Geometry: final body of the model. Coordinates: model frame, mm. A direction names the side the tool comes from. Give positions to 0.01 mm unless a question says otherwise; leave off trailing zeros. Order: outer loops, then holes, each group sorted by start corner. A loop starts at its lowest first (then second) coordinate and runs counter-clockwise, first axis right, second up. Notation, with made-up numbers: (-39, 23) -> (16, 23) arc R20 ccw to (16, 30) -> close; hole circle Ø3 at (14.5, -15.75). An arc over 180 degrees is marked (long way). One line per item, written item: value. Start each with the question number.
```python
from build123d import *

# Parameters (mm, degrees)
EXTRUDE_1_DEPTH     = 60
SKETCH_3_R          = 2.3
CUT_EXTRUDE_1_DEPTH = 30
SKETCH_4_W          = 30
SKETCH_4_H          = 50
EXTRUDE_2_DEPTH     = 3
EXTRUDE_3_DEPTH     = 15
SKETCH_6_W          = 47.657493386
SKETCH_6_H          = 61.593201797
CUT_EXTRUDE_2_DEPTH = 30
SKETCH_7_R          = 3.2
CUT_EXTRUDE_3_DEPTH = 3


with BuildPart() as part:
    # 草图2 → 凸台-拉伸1 (new body)
    with BuildSketch(Plane(origin=(0, 0, 0), x_dir=(1, 0, 0), z_dir=(0, 1, 0))):
        with BuildLine():
            Line((-4, 6), (4, 6))
            ThreePointArc((4, 6), (10, 0), (4, -6))
            Line((4, -6), (-4, -6))
            ThreePointArc((-4, -6), (-10, 0), (-4, 6))
        make_face()
        with BuildLine():
            Line((-2.5, 4.05), (2.5, 4.05))
            ThreePointArc((2.5, 4.05), (6.55, 0), (2.5, -4.05))
            Line((2.5, -4.05), (-2.5, -4.05))
            ThreePointArc((-2.5, -4.05), (-6.55, 0), (-2.5, 4.05))
        make_face(mode=Mode.SUBTRACT)
    extrude(amount=EXTRUDE_1_DEPTH)

    # 草图3 → 切除-拉伸1 (cut)
    with BuildSketch(Plane.XY.offset(6)):
        with Locations((0, 55.049214592)):
            Circle(SKETCH_3_R)
        with Locations((0, 45.049214592)):
            Circle(SKETCH_3_R)
        with Locations((0, 35.049214592)):
            Circle(SKETCH_3_R)
        with Locations((0, 25.049214592)):
            Circle(SKETCH_3_R)
        with Locations((0, 15.049214592)):
            Circle(SKETCH_3_R)
        with Locations((0, 5.049214592)):
            Circle(SKETCH_3_R)
    extrude(amount=-CUT_EXTRUDE_1_DEPTH, mode=Mode.SUBTRACT)

    # 草图4 → 凸台-拉伸2 (add)
    with BuildSketch(Plane.XZ):
        Rectangle(SKETCH_4_W, SKETCH_4_H)
    extrude(amount=EXTRUDE_2_DEPTH)

    # 草图5 → 凸台-拉伸3 (add, symmetric)
    with BuildSketch(Plane(origin=(0, 0, 0), x_dir=(0, 0, -1), z_dir=(1, 0, 0))):
        Polygon((-25, -3), (-21, -3), (-21, -6), (-9, -6), (-9, -9), (-25, -9), (-25, -6), align=None)
        Polygon((25, -3), (21, -3), (21, -6), (9, -6), (9, -9), (25, -9), (25, -6), align=None)
    extrude(amount=EXTRUDE_3_DEPTH, both=True)

    # 草图6 → 切除-拉伸2 (cut)
    with BuildSketch(Plane(origin=(0, 0, 0), x_dir=(1, 0, 0), z_dir=(0, 1, 0))):
        with Locations((1.592624165, 0.101186893)):
            Rectangle(SKETCH_6_W, SKETCH_6_H)
        with BuildLine():
            Line((15, -19), (15, 19))
            ThreePointArc((15, 19), (13.242640687, 23.242640687), (9, 25))
            Line((9, 25), (-9, 25))
            ThreePointArc((-9, 25), (-13.242640687, 23.242640687), (-15, 19))
            Line((-15, 19), (-15, -19))
            ThreePointArc((-15, -19), (-13.242640687, -23.242640687), (-9, -25))
            Line((-9, -25), (9, -25))
            ThreePointArc((9, -25), (13.242640687, -23.242640687), (15, -19))
        make_face(mode=Mode.SUBTRACT)
    extrude(amount=-CUT_EXTRUDE_2_DEPTH, mode=Mode.SUBTRACT)

    # 草图7 → 切除-拉伸3 (cut)
    with BuildSketch(Plane(origin=(0, 0, 0), x_dir=(1, 0, 0), z_dir=(0, 1, 0))):
        with Locations(Location((0, 14, 0), (0, 0, 270))):
            Circle(SKETCH_7_R)
        with Locations(Location((0, -14, 0), (0, 0, 90))):
            Circle(SKETCH_7_R)
    extrude(amount=-CUT_EXTRUDE_3_DEPTH, mode=Mode.SUBTRACT)


solid = part.part
```
1. Cut plane B-B, the plane z = 0. Return loops of the section in (x, y).
2. Cut plane C-C, the plane x = 11. Return loops of the section in (y, z), then the cut area to 3 significant figures.
3. Draft query along Z for faces 4 (the cylindrical face through (-10, 30, 0)), 5 (the flat face through (0, 30, -4.05)), 6 (the flat face through (-7, 0, 6)). Return one class per face: pulls with the +Z half, pulls with the -Z half, needs draft (parallel to the pull), parting line crosses it, or undercut.
4. Pin query (flat end, axial travel): P1, Ø4, axis at x = 0, y = 45.05, coming from the +Z side; P2, Ø5, axis at x = 0, z = 14, coming from the +Y side; P3, Ø5.5, axis at x = 0, y = 15.05, coming from the +Z side; P4, Ø5, axis at x = -11, y = 11.5, coming from the -Z side. Return the tip coordinate at first contact, or that it passes through.
5. Material intervals for L1, parallel to Z at x = 7.5, y = -5.5; L2, parallel to Y at x = 12, z = -14; L3, parallel to X at y = -1, z = -14, sorted ascending. Write a range as [from, to].
6. Access query for faces 1 (the flat face through (0, -7, -9)), 2 (the flat face through (0, 30, -6)), 3 (the flat face through (0, -3, 0)). Directions: +Z, -Z, +X, -X, +Y, -Y. A direction counts if a zero-diameter tool reaches every point of the face in a straight line with its end or side. Return the directions, or none.
7. Cut plane A-A, the plane z = -14. Return loops of the section in (x, y), then the cut area to 3 significant figures.
8. Cut plane D-D, the plane x = 0. State how many separate pieces and enclosed holes the cut face has, then the cut area to 3 significant figures.
Answers follow:
1. outline: (-15, -3) -> (15, -3) -> (15, 0) -> (10, 0) -> (10, 60) -> (6.55, 60) -> (6.55, 0) -> (-6.55, 0) -> (-6.55, 60) -> (-10, 60) -> (-10, 0) -> (-15, 0) -> close
2. outline: (-9, -24.66) -> (0, -24.66) -> (0, 24.66) -> (-9, 24.66) -> (-9, 9) -> (-6, 9) -> (-6, 21) -> (-3, 21) -> (-3, -21) -> (-6, -21) -> (-6, -9) -> (-9, -9) -> close
2. area: 264 mm²
3. face 4: parting line crosses it
3. face 5: undercut
3. face 6: needs draft
4. P1: passes through
4. P2: stops at y = -6
4. P3: stops at z = 6
4. P4: stops at z = -3.97
5. L1: z = [-25, -21], [21, 25]
5. L2: y = [-9, -6], [-3, 0]
5. L3: x = [-15, -3.2], [3.2, 15]
6. face 1: +X, -X, -Y
6. face 2: -Z, +X, -X, +Y
6. face 3: +X, -X
7. outline: (-15, -9) -> (15, -9) -> (15, -6) -> (-15, -6) -> close; (-15, -3) -> (-3.2, -3) -> (-3.2, 0) -> (-15, 0) -> close; (3.2, -3) -> (15, -3) -> (15, 0) -> (3.2, 0) -> close
7. area: 161 mm²
8. separate pieces: 15
8. enclosed holes: 0
8. area: 358 mm²
